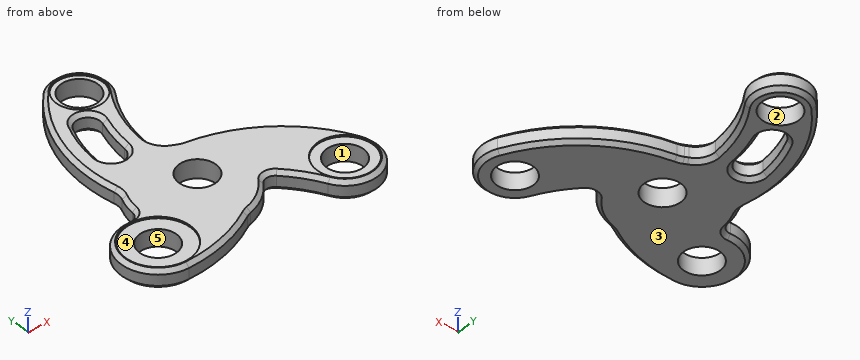
from build123d import *

# Parameters (mm, degrees)
F1_R      = 6.35
F2_DEPTH  = 3.175
F3_R      = 6.35
F4_DEPTH  = 6.351
F5_R      = 6.35
F6_R      = 3.175
F7_R      = 11.1125
F7_R_2    = 9.525
F7_R_3    = 7.9375
F8_DEPTH  = 0.53975
F11_DEPTH = 25.4
F12_SIZE  = 1.3335


with BuildPart() as f2:
    # F1 (on Top) → F2 (new body, symmetric)
    with BuildSketch(Plane.XY):
        with BuildLine():
            ThreePointArc((-0.168710733, 16.2535201518), (1.7967030303, 29.8395650927), (7.8138383534, 42.1780232985))
            ThreePointArc((7.8138383534, 42.1780232985), (6.1225519823, 54.9215733207), (-6.7210836767, 54.3742710132))
            ThreePointArc((-6.7210836767, 54.3742710132), (-19.6290735416, 32.6508588295), (-20.4740110981, 7.3959797012))
            ThreePointArc((-20.4740110981, 7.3959797012), (-22.6457174108, 2.0757674769), (-23.1321493543, -3.6499945148))
            ThreePointArc((-23.1321493543, -3.6499945148), (-24.3075600188, -3.5087608054), (-25.4787925595, -3.3362744979))
            ThreePointArc((-25.4787925595, -3.3362744979), (-40.1479792359, -14.7681220671), (-27.6867699643, -28.5735717187))
            ThreePointArc((-27.6867699643, -28.5735717187), (-13.4568579615, -26.7614387597), (-0.300857561, -21.0435829613))
            ThreePointArc((-0.300857561, -21.0435829613), (7.8163915703, -17.2243931464), (13.2856838039, -10.1136416555))
            ThreePointArc((13.2856838039, -10.1136416555), (19.5634681844, -16.7944756929), (24.337196584, -24.6210737617))
            ThreePointArc((24.337196584, -24.6210737617), (39.0667286463, -29.9150952834), (44.4792335839, -15.2286876578))
            ThreePointArc((44.4792335839, -15.2286876578), (28.8065675228, 4.269400985), (5.72810807, 13.9230340561))
            ThreePointArc((5.72810807, 13.9230340561), (2.8773398413, 15.3353381376), (-0.168710733, 16.2535201518))
        make_face()
        Circle(F1_R, mode=Mode.SUBTRACT)
    extrude(amount=F2_DEPTH, both=True)

    # F3 (on face) → F4 (cut, through all)
    with BuildSketch(Plane.XY.offset(3.175)):
        with Locations((0, 47.625)):
            Circle(F3_R)
        with Locations((34.3703832127, -19.84375)):
            Circle(F3_R)
        with Locations((-27.4963065702, -15.875)):
            Circle(F3_R)
    extrude(amount=-F4_DEPTH, mode=Mode.SUBTRACT)

    # F5
    f5_edges = [f2.edges().sort_by_distance(p)[0] for p in [
        (-20.474011, 7.39598, 0),
        (-0.168711, 16.25352, 0),
        (5.728108, 13.923034, 0),
        (-0.300858, -21.043583, 0),
    ]]
    fillet(f5_edges, radius=F5_R)

    # F6
    f6_edges = [f2.edges().sort_by_distance(p)[0] for p in [
        (13.285684, -10.113642, 0),
        (-23.132149, -3.649995, 0),
    ]]
    fillet(f6_edges, radius=F6_R)

    # F7 (on face) → F8 (cut)
    with BuildSketch(Plane.XY.offset(3.175)):
        with Locations((-27.4963065702, -15.875)):
            Circle(F7_R)
        with Locations((34.3703832127, -19.84375)):
            Circle(F7_R_2)
        with Locations((0, 47.625)):
            Circle(F7_R_3)
    extrude(amount=-F8_DEPTH, mode=Mode.SUBTRACT)

    # F10 (on face) → F11 (cut)
    with BuildSketch(Plane.XY.offset(3.175)):
        with BuildLine():
            ThreePointArc((-10.9775403861, 37.5513992072), (-13.6403456115, 30.5006059619), (-15.0736581613, 23.1012930078))
            ThreePointArc((-15.0736581613, 23.1012930078), (-11.1261361584, 18.2091441919), (-6.2339873425, 22.1566661948))
            ThreePointArc((-6.2339873425, 22.1566661948), (-5.1843883194, 28.3376957326), (-3.3814010551, 34.3423623497))
            ThreePointArc((-3.3814010551, 34.3423623497), (-5.6475239326, 39.5731654756), (-10.9775403861, 37.5513992072))
        make_face()
    extrude(amount=-F11_DEPTH, mode=Mode.SUBTRACT)

    # F12
    f12_edges = [f2.edges().sort_by_distance(p)[0] for p in [
        (-13.91632, -26.88546, 3.175),
        (-13.91632, -26.88546, -3.175),
        (-13.640346, 30.500606, 3.175),
        (-5.647524, 39.573165, -3.175),
    ]]
    chamfer(f12_edges, length=F12_SIZE)


solid = f2.part
The model under review builds one solid part; all positions refer to its coordinate system, in mm. Face numbers are marked on the shaded views. A direction names the side the tool comes from. Round coordinates to 2 decimals unless told otherwise and drop trailing zeros. Answer as a JSON object with one key per item and string values.
Item 1: For line 1 along X through (y, z) = (31, -2.25); line 2 along X through (y, z) = (30.5, 2); line 3 along Y through (x, z) = (-8, -1.75), list the stretches that pass through material, from the lowest coordinate up.
Check sheet entries:
{"line 1": "-19.66 to -13.92, -4.06 to 1.74", "line 2": "-20.04 to -13.81, -4.46 to 1.84", "line 3": "-24.92 to 19.06, 39.83 to 53.05"}
Item 2: Clearance check with flat-ended pins moving along their axes: P1, Ø7.5, axis at x = 0, y = 0, coming from the +Z side; P2, Ø2, axis at x = 12.5, z = 2.5, coming from the +Y side; P3, Ø3, axis at y = 6.5, z = -1.5, coming from the -X side. State where each tip first meets the part, or that it passes through.
Check sheet entries:
{"P1": "through", "P2": "y = 12.65", "P3": "x = -21.69"}
Item 3: The part is to be moulded in two halves that separate along Y. For the marked faces 1, 2 and 3, say which applies: +Y half, -Y half, draft (parallel to the pull), parting line (faces both ways), or undercut.
Check sheet entries:
{"face 1": "undercut", "face 2": "undercut", "face 3": "draft"}
Item 4: Tool access review of the marked faces 4 and 5: name each direction out of +Z, -Z, +X, -X, +Y, -Y from which nothing blocks a thin tool from reaching the whole face with its end or side.
Check sheet entries:
{"face 4": "+Z", "face 5": "+Z, -Z"}
